Source: CAD feature listing. Evaluate the final solid. Frame: model axes, mm. A direction names the side the tool comes from. Round coordinates to 2 decimals unless told otherwise and drop trailing zeros. Loops run counter-clockwise (first coordinate to the right, second up) from the corner with the lowest first, then second, coordinate; pieces in that order, holes last. Notation, with made-up numbers: (-22, 26.5) -> (36, 26.5) arc R11 cw to (36, 33.5) -> close; hole circle Ø1 at (-31, 49.5). An arc over 180 degrees is marked (long way). Write item = value, one per line.
from build123d import *

# Parameters (mm, degrees)
SKETCH1_W           = 32
SKETCH1_H           = 27
BOSS_EXTRUDE1_DEPTH = 10
FILLET1_R           = 2
CUT_EXTRUDE4_DEPTH  = 26
SKETCH4_R           = 3
BOSS_EXTRUDE2_DEPTH = 18
FILLET2_R           = 2


with BuildPart() as part:
    # Sketch1 → Boss-Extrude1 (new body)
    with BuildSketch(Plane.XY):
        Rectangle(SKETCH1_W, SKETCH1_H)
    extrude(amount=BOSS_EXTRUDE1_DEPTH)

    # Fillet1
    fillet1_edges = [part.edges().sort_by_distance(p)[0] for p in [
        (-16, -13.5, 5),
        (16, -13.5, 5),
        (16, 13.5, 5),
        (-16, 13.5, 5),
    ]]
    fillet(fillet1_edges, radius=FILLET1_R)

    # Sketch2 → Cut-Extrude4 (cut)
    with BuildSketch(Plane(origin=(0, 13.5, 0), x_dir=(1, 0, 0), z_dir=(0, 1, 0))):
        Polygon((-9, -10), (-9, -8), (-11, -8), (-11, -5), (11, -5), (11, -8), (9, -8), (9, -10), align=None)
    extrude(amount=-CUT_EXTRUDE4_DEPTH, mode=Mode.SUBTRACT)

    # Sketch4 → Boss-Extrude2 (add)
    with BuildSketch(Plane(origin=(0, 0, 0), x_dir=(-1, 0, 0), z_dir=(0, 0, -1))):
        Circle(SKETCH4_R)
    extrude(amount=BOSS_EXTRUDE2_DEPTH)

    # Fillet2
    fillet2_edges = [part.edges().sort_by_distance(p)[0] for p in [
        (3, 0, 0),
    ]]
    fillet(fillet2_edges, radius=FILLET2_R)


solid = part.part
1. Mould query, pull axis X, two halves, no side actions, for faces 6 (the face through (0, 1, 5)), 7 (the face through (-10, 1, 8)), 8 (the face through (-15.43, 12.9, 5.07)), 9 (the face through (-11, 0, 10)). Classes: released by +X, released by -X, zero draft, split by the parting line, or undercut.
Evaluation:
face_6 = undercut
face_7 = undercut
face_8 = released by -X
face_9 = zero draft
2. Contact query for flat-ended pins moving along their axis: pin 1 Ø1 at (x, y) = (0.5, 4.5) entering from +Z; pin 2 Ø2 at (y, z) = (5.5, -3.5) entering from +X; pin 3 Ø1.5 at (x, z) = (-5, 6.5) entering from +Y; pin 4 Ø1.6 at (x, y) = (-10, 2) entering from -Z. Output: stop coordinate, or through.
Evaluation:
pin_1 = 5
pin_2 = through
pin_3 = -12.5
pin_4 = 0
3. Line query: probe 1 along Z at (x, y) = (-10, 12.25); probe 2 along Z at (x, y) = (14, 12.5); probe 3 along Z at (x, y) = (3, -6). Output: solid intervals per line, ascending. Write a range as from..to.
Evaluation:
probe_1 = 0..5, 8..10
probe_2 = 0..10
probe_3 = 0..5
4. Section query C-C (y = -11). Return the cut outline in (x, z).
Evaluation:
outline = (-16, 0) -> (16, 0) -> (16, 10) -> (9, 10) -> (9, 8) -> (11, 8) -> (11, 5) -> (-11, 5) -> (-11, 8) -> (-9, 8) -> (-9, 10) -> (-16, 10) -> close
5. Set-up query: faces 1 (the face through (0, 0, -18)), 2 (the face through (16, 0, 5)), 3 (the face through (-9, 1, 9)), 4 (the face through (-11, 1, 7)), 5 (the face through (3, 0, -10)). Return all of +Z, -Z, +X, -X, +Y, -Y with unobstructed straight access to the full face (end or side cutting, diameter ignored); none if empty.
Evaluation:
face_1 = -Z, +X, -X, +Y, -Y
face_2 = +Z, -Z, +X, +Y, -Y
face_3 = +Z, +Y
face_4 = +Y
face_5 = -Z
6. Section query B-B (x = 6). Return the cut outline in (y, z).
Evaluation:
outline = (-13.5, 0) -> (13.5, 0) -> (13.5, 5) -> (-12.5, 5) -> (-12.5, 10) -> (-13.5, 10) -> close
7. Section query D-D (z = -3). Return the cut outline in (x, y), then the cut area to 3 significant figures.
Evaluation:
outline = circle Ø6 at (0, 0)
area = 28.3 mm²
8. Section query A-A (y = 0). Return the cut outline in (x, z).
Evaluation:
outline = (-16, 0) -> (-5, 0) arc R2 cw to (-3, -2) -> (-3, -18) -> (3, -18) -> (3, -2) arc R2 cw to (5, 0) -> (16, 0) -> (16, 10) -> (9, 10) -> (9, 8) -> (11, 8) -> (11, 5) -> (-11, 5) -> (-11, 8) -> (-9, 8) -> (-9, 10) -> (-16, 10) -> close
